For this review, take the finished solid that the model builds, in its own axes (mm). Give positions to 0.01 mm unless a question says otherwise; leave off trailing zeros. Order: outer loops, then holes, each group sorted by start corner. A loop starts at its lowest first (then second) coordinate and runs counter-clockwise, first axis right, second up.
Item 1: The part is to be moulded in two halves that separate along X. For faces 1 (the cylindrical face through (-4.46, 0.59, 3.21)), 2 (the cylindrical face through (5.96, -1.88, 5.49)), 3 (the flat face through (-2, 5, 6.5)), 4 (the flat face through (7, 0, 2)), say which applies: released by +X, released by -X, zero draft, split by the parting line, or undercut.
Item 2: Consider section C-C (z = 5.75). Give the boundary of the cut face in (x, y).
Item 3: For probe 1 along X at (y, z) = (0, 3); probe 2 along X at (y, z) = (-0.5, 6.25); probe 3 along Z at (x, y) = (-6, 4.25), list the stretches that pass through material, from the lowest coordinate up.
Item 4: Consider section A-A (y = 0). Give the boundary of the cut face in (x, z), plus the area to 3 significant figures.
Item 5: For P1, Ø1, axis at x = 4.5, z = 4.5, coming from the -Y side; P2, Ø4, axis at x = 2.5, y = 2.5, coming from the +Z side; P3, Ø1.5, axis at y = 6, z = 3.5, coming from the -X side; P4, Ø1.5, axis at x = 4, z = 2, coming from the +Y side, all flat-tipped, find the tip position at first contact; note any pin that passes through.
Item 6: Consider section B-B (z = 3.25). Give the boundary of the cut face in (x, y).
Autodesk Inventor part; units mm, degrees
ref_plane "Piano di lavoro1" through (0, 0, 2) normal (0, 0, -1) x (-1, 0, 0)
ref_plane "YZ Plane" through (0, 0, 0) normal (1, 0, 0) x (0, 1, 0)
ref_plane "XZ Plane" through (0, 0, 0) normal (0, 1, 0) x (-1, 0, 0)
sketch "Schizzo1" plane through (0, 0, 0) normal (0, 0, 1) x (1, 0, 0)
  line L0 (0, 8.0829) -> (7, 4.0415)
  line L1 (7, 4.0415) -> (7, -4.0415)
  line L2 (7, -4.0415) -> (0, -8.0829)
  line L3 (0, -8.0829) -> (-7, -4.0415)
  line L4 (-7, -4.0415) -> (-7, 4.0415)
  line L5 (-7, 4.0415) -> (0, 8.0829)
  point P0 (0, 0)
  point P1 (0, 0)
  dimension "d0" = 14
extrude "Estrusione1" add sketch "Schizzo1" along normal blind 5
sketch "Schizzo2" plane through (0, 0, 5) normal (0, 0, 1) x (1, 0, 0)
  circle A0 centre (0, 0) radius 6.25
  dimension "d5" = 12.5
extrude "Estrusione2" add sketch "Schizzo2" along normal blind 1.5
sketch "Schizzo3" plane through (0, 0, 0) normal (1, 0, 0) x (0, 1, 0)
  line L0 (8.0829, 5) -> (4.0415, 5)
  line L1 (4.0415, 0) -> (4.0415, 5)
  line L2 (8.0829, 0) -> (4.0415, 0)
  line L3 (8.0829, 0) -> (8.0829, 5)
  line L4 (6.4929, 0) -> (8.0829, 0.918)
  line L5 (0, -0.8) -> (0, 4.8)
  line L6 (6.4929, 5) -> (8.0829, 4.082)
  line L7 (6.4929, 5) -> (8.0829, 5)
  line L8 (8.0829, 4.082) -> (8.0829, 5)
  point P0 (0, 0)
  dimension "d6" = 30
ref_plane "Piano di lavoro1" through (0, 0, 2) normal (0, 0, -1) x (-1, 0, 0)
sketch "Schizzo4" plane through (0, 0, 6.5) normal (0, 0, 1) x (1, 0, 0)
  circle A0 centre (0, 0) radius 6.25
hole "Foro1" at (0, 0, 6.5) direction (0, 0, -1) diameter 9 end through all
thread "Filettatura1"
chamfer "Smusso1" distance 0.5 angle 45 2 edges at (0, 4.5, 6.5) (0, 4.5, 0)
revolve "Rivoluzione2" cut sketch "Schizzo3" angle 360 about axis through (0, 0, -10) along (0, 0, 1) contours L3 L6 L0 | L3 L2 L4
fillet "Raccordo1" radius 0.5 1 edges at (-6.25, 0, 6.5)
properties part number "Dado 14"
Resolved:
1. face 1: undercut
1. face 2: split by the parting line
1. face 3: zero draft
1. face 4: released by +X
2. outline: circle Ø12.5 at (0, 0); hole circle Ø9 at (0, 0)
3. probe 1: x = -7 to -4.5, 4.5 to 7
3. probe 2: x = -6.16 to -4.72, 4.72 to 6.16
3. probe 3: z = 0.5 to 4.5
4. outline: (-7, 0.29) - (-6.49, 0) - (-5, 0) - (-4.5, 0.5) - (-4.5, 6) - (-5, 6.5) - (-5.75, 6.5) arc R0.5 ccw to (-6.25, 6) - (-6.25, 5) - (-6.49, 5) - (-7, 4.71) - close; (4.5, 0.5) - (5, 0) - (6.49, 0) - (7, 0.29) - (7, 4.71) - (6.49, 5) - (6.25, 5) - (6.25, 6) arc R0.5 ccw to (5.75, 6.5) - (5, 6.5) - (4.5, 6) - close
4. area: 29.3 mm2
5. P1: stops at y = -5.77
5. P2: stops at z = 6.5
5. P3: stops at x = -4.91
5. P4: stops at y = 6.21
6. outline: (-7, -4.04) - (0, -8.08) - (7, -4.04) - (7, 4.04) - (0, 8.08) - (-7, 4.04) - close; hole circle Ø9 at (0, 0)
